Here's how the part is built. I have some questions about the finished solid (model axes, mm). A direction names the side the tool comes from. Round coordinates to 2 decimals unless told otherwise and drop trailing zeros. Write each loop counter-clockwise with the first axis right and the second up, starting at its lowest first coordinate (ties: lowest second). Pieces come first, ordered by that corner, then holes. Notation, with made-up numbers: M -1,-9 L 35,-9 A14 cw 35,8 Z; hole C 40.25,38.5 d7. An arc over 180 degrees is marked long. Use a Markdown table: item, result. Add a question column.
```python
from build123d import *

# Parameters (mm, degrees)
SKETCH1_W                                 = 60
SKETCH1_H                                 = 120
BOSS_EXTRUDE1_DEPTH                       = 12.7
SKETCH2_W                                 = 34.6
SKETCH2_H                                 = 7.7
CUT_EXTRUDE1_DEPTH                        = 121
F_3_32_0_09375_DIAMETER_HOLE3_D           = 2.38125
F_3_32_0_09375_DIAMETER_HOLE3_DEPTH       = 19.05
F_3_32_0_09375_DIAMETER_HOLE3_CSINK_D     = 3.175
F_3_32_0_09375_DIAMETER_HOLE3_CSINK_ANGLE = 90
F_3_32_0_09375_DIAMETER_HOLE3_TIP         = 0.715399675
CUT_EXTRUDE2_DEPTH                        = 1
CUT_EXTRUDE2_DEPTH_BACK                   = 121
F_5_16_18_TAPPED_HOLE1_D                  = 6.5278
F_5_16_18_TAPPED_HOLE1_DEPTH              = 32.45
F_5_16_18_TAPPED_HOLE1_CSINK_D            = 9.2075
F_5_16_18_TAPPED_HOLE1_CSINK_ANGLE        = 90
F_5_16_18_TAPPED_HOLE1_TIP                = 1.961148974
CHAMFER1_SIZE                             = 3.175
SKETCH7_R                                 = 4
CUT_EXTRUDE4_DEPTH                        = 6
CHAMFER2_SIZE                             = 2
SKETCH10_W                                = 60
SKETCH10_H                                = 100.95
CUT_EXTRUDE5_DEPTH                        = 7.7
SKETCH11_W                                = 24.87086649
SKETCH11_H                                = 0.4
CUT_EXTRUDE6_DEPTH                        = 121.0000001
SKETCH12_W                                = 34.6
SKETCH12_H                                = 0.374910819
CUT_EXTRUDE7_DEPTH                        = 121


with BuildPart() as part:
    # Sketch1 → Boss-Extrude1 (new body)
    with BuildSketch(Plane(origin=(0, 0, 0), x_dir=(1, 0, 0), z_dir=(0, 1, 0))):
        with Locations((0, 60)):
            Rectangle(SKETCH1_W, SKETCH1_H)
    extrude(amount=BOSS_EXTRUDE1_DEPTH)

    # Sketch2 → Cut-Extrude1 (cut, through all)
    with BuildSketch(Plane.XY):
        with Locations((0, 8.85)):
            Rectangle(SKETCH2_W, SKETCH2_H)
    extrude(amount=-CUT_EXTRUDE1_DEPTH, mode=Mode.SUBTRACT)

    # 3_32 _0.09375_ Diameter Hole3
    with Locations(Plane.XY):
        with Locations((0, 2.61875)):
            CounterSinkHole(F_3_32_0_09375_DIAMETER_HOLE3_D / 2, F_3_32_0_09375_DIAMETER_HOLE3_CSINK_D / 2, depth=F_3_32_0_09375_DIAMETER_HOLE3_DEPTH, counter_sink_angle=F_3_32_0_09375_DIAMETER_HOLE3_CSINK_ANGLE)
            with Locations((0, 0, -(F_3_32_0_09375_DIAMETER_HOLE3_DEPTH + F_3_32_0_09375_DIAMETER_HOLE3_TIP / 2))):  # 118° drill point
                Cone(0, F_3_32_0_09375_DIAMETER_HOLE3_D / 2, F_3_32_0_09375_DIAMETER_HOLE3_TIP, mode=Mode.SUBTRACT)

    # Sketch3 → Cut-Extrude2 (cut, two sides)
    with BuildSketch(Plane.XY) as cut_extrude2_sk:
        with BuildLine():
            Line((-124.818289263, -9.651397294), (-17.3, 0))
            ThreePointArc((-17.3, 0), (0, 0.774910819), (17.3, 0))
            Line((17.3, 0), (124.818289263, -9.651397294))
            Line((124.818289263, -9.651397294), (124.818289263, -225.552596882))
            Line((124.818289263, -225.552596882), (-124.818289263, -225.552596882))
            Line((-124.818289263, -225.552596882), (-124.818289263, -9.651397294))
        make_face()
    extrude(amount=CUT_EXTRUDE2_DEPTH, mode=Mode.SUBTRACT)
    extrude(cut_extrude2_sk.sketch, amount=-CUT_EXTRUDE2_DEPTH_BACK, mode=Mode.SUBTRACT)

    # 5_16-18 Tapped Hole1
    with Locations(Plane.XY):
        with Locations((-23.65, 6.35), (23.65, 6.35)):
            CounterSinkHole(F_5_16_18_TAPPED_HOLE1_D / 2, F_5_16_18_TAPPED_HOLE1_CSINK_D / 2, depth=F_5_16_18_TAPPED_HOLE1_DEPTH, counter_sink_angle=F_5_16_18_TAPPED_HOLE1_CSINK_ANGLE)
            with Locations((0, 0, -(F_5_16_18_TAPPED_HOLE1_DEPTH + F_5_16_18_TAPPED_HOLE1_TIP / 2))):  # 118° drill point
                Cone(0, F_5_16_18_TAPPED_HOLE1_D / 2, F_5_16_18_TAPPED_HOLE1_TIP, mode=Mode.SUBTRACT)

    # Chamfer1
    chamfer1_edges = [part.edges().sort_by_distance(p)[0] for p in [
        (-17.3, 12.7, -60),
        (17.3, 12.7, -60),
    ]]
    chamfer(chamfer1_edges, length=CHAMFER1_SIZE)

    # Sketch7 → Cut-Extrude4 (cut, through all)
    with BuildSketch(Plane(origin=(0, 5, 0), x_dir=(1, 0, 0), z_dir=(0, 1, 0))):
        with Locations(Location((5, 107.9216, 0), (0, 0, 270))):  # turned: the seam where the file's is
            Circle(SKETCH7_R)
        with Locations(Location((-1.2489, 47.6216, 0), (0, 0, 270))):  # turned: the seam where the file's is
            Circle(SKETCH7_R)
    extrude(amount=-CUT_EXTRUDE4_DEPTH, mode=Mode.SUBTRACT)

    # Chamfer2
    chamfer2_edges = [part.edges().sort_by_distance(p)[0] for p in [
        (5, 5, -111.9216),
        (-1.2489, 5, -51.6216),
    ]]
    chamfer(chamfer2_edges, length=CHAMFER2_SIZE)

    # Sketch10 → Cut-Extrude5 (cut)
    with BuildSketch(Plane(origin=(0, 12.7, 0), x_dir=(1, 0, 0), z_dir=(0, 1, 0))):
        with Locations((0, 69.525)):
            Rectangle(SKETCH10_W, SKETCH10_H)
    extrude(amount=-CUT_EXTRUDE5_DEPTH, mode=Mode.SUBTRACT)

    # Sketch11 → Cut-Extrude6 (cut, through all)
    with BuildSketch(Plane.XY):
        with Locations((0, 0.574910819)):
            Rectangle(SKETCH11_W, SKETCH11_H)
    extrude(amount=-CUT_EXTRUDE6_DEPTH, mode=Mode.SUBTRACT)

    # Sketch12 → Cut-Extrude7 (cut, through all)
    with BuildSketch(Plane.XY):
        with Locations((0, 0.18745541)):
            Rectangle(SKETCH12_W, SKETCH12_H)
    extrude(amount=-CUT_EXTRUDE7_DEPTH, mode=Mode.SUBTRACT)


solid = part.part
```
Item 1: Imagine slicing it at A-A on x = -23.65. List the corners of the cut face in (y, z) for me, plus the area to 3 significant figures.
Item 2: On a 3-axis mill with a long thin cutter (end or side, diameter ignored), from which of +Z, -Z, +X, -X, +Y, -Y can I reach the whole of each face in a straight line? I mean faces 1 (the face through (0, 0.775, -59)), 2 (the face through (17.3, 7, -9)), 3 (the face through (-0.4, 4.8, 0)), 4 (the face through (-22.942, 3.164, -13.656)), 5 (the face through (-24, 10, -19.05)). Say none if no direction works.
Item 3: Imagine slicing it at B-B on z = -66.5. List the corners of the cut face in (x, y) for me.
Item 4: For pin 1 Ø6 at (x, y) = (-11, 6.5) entering from +Z; pin 2 Ø6 at (x, y) = (5.5, 9.5) entering from +Z; pin 3 Ø9 at (x, z) = (5, -107.92) entering from -Y; pin 4 Ø4 at (x, y) = (26, 10) entering from -Z, each with a flat end and sliding along its axis, tell me the tip position at first contact or that it passes through.
Item 5: Imagine slicing it at C-C on z = -17.5. List the corners of the cut face in (x, y) for me (3 decimals), plus the area to 3 significant figures.
Item 6: I need wall thicknesses on probe 1 along X at (y, z) = (6.35, -8.5); probe 2 along Y at (x, z) = (0, -4); probe 3 along Z at (x, y) = (21.5, 10.75). Which ranges of each line are inside material? Lowest first, please. Write a range as from..to.
Item 7: Imagine slicing it at D-D on y = 7.5. Count the separate pieces of the cut face and the enclosed holes in it, plus the area to 3 significant figures.
Item 8: If we mould it in two halves opening along Y, with no side actions, what happens to faces 6 (the face through (25, 12.7, -10)), 7 (the face through (-30, 3, -59)), 8 (the face through (24.358, 3.164, -13.656))? For each: +Y half, -Y half, draft (parallel to the pull), parting line (faces both ways), or undercut.
The answers:
| question | item | result |
|---|---|---|
| 1 | outline | M 0,-120 L 5,-120 L 5,-33.6 L 3.09,-32.45 L 3.09,-1.34 L 1.75,0 L 0,0 Z; M 9.61,-19.05 L 12.7,-19.05 L 12.7,0 L 10.95,0 L 9.61,-1.34 Z |
| 1 | area | 594 mm² |
| 2 | face 1 | +Z, -Z, -Y |
| 2 | face 2 | +Z, -Z, +Y |
| 2 | face 3 | +Z, +X, -X, +Y, -Y |
| 2 | face 4 | +Z |
| 2 | face 5 | -Z, +X, -X, +Y |
| 3 | outline | M -30,0 L -17.3,0 L -17.3,0.37 L -12.44,0.37 L -12.44,0.77 L 12.44,0.77 L 12.44,0.37 L 17.3,0.37 L 17.3,0 L 30,0 L 30,5 L -30,5 Z |
| 4 | pin 1 | z = 0 |
| 4 | pin 2 | through |
| 4 | pin 3 | y = 0.77 |
| 4 | pin 4 | z = -19.05 |
| 5 | outline | M -30,0 L -17.3,0 L -17.3,0.375 L -12.435,0.375 L -12.435,0.775 L 12.435,0.775 L 12.435,0.375 L 17.3,0.375 L 17.3,0 L 30,0 L 30,12.7 L 20.475,12.7 L 17.3,9.525 L 17.3,5 L -17.3,5 L -17.3,9.525 L -20.475,12.7 L -30,12.7 Z; hole C -23.65,6.35 d6.528; hole C 0,2.619 d2.381; hole C 23.65,6.35 d6.528 |
| 5 | area | 391 mm² |
| 6 | probe 1 | -30..-26.91, -20.39..-17.3, 17.3..20.39, 26.91..30 |
| 6 | probe 2 | 0.77..1.43, 3.81..5 |
| 6 | probe 3 | -19.05..0 |
| 7 | separate pieces | 4 |
| 7 | enclosed holes | 0 |
| 7 | area | 247 mm² |
| 8 | face 6 | +Y half |
| 8 | face 7 | draft |
| 8 | face 8 | undercut |
